Part print with two shaded views. Sizes in mm from the minimum x, y, z corner. A direction names the side the tool comes from. Coordinates: 2 decimals unless noted, no trailing zeros. Loops run counter-clockwise (first coordinate to the right, second up) from the corner with the lowest first, then second, coordinate; pieces in that order, holes last. Notation, with made-up numbers: (47.5, 21.5) -> (83.5, 21.5) arc R20 cw to (83.5, 55.5) -> close; hole circle Ø7 at (27.25, -16). An arc over 180 degrees is marked (long way). One line per item, written item: value. Start each with the question number.
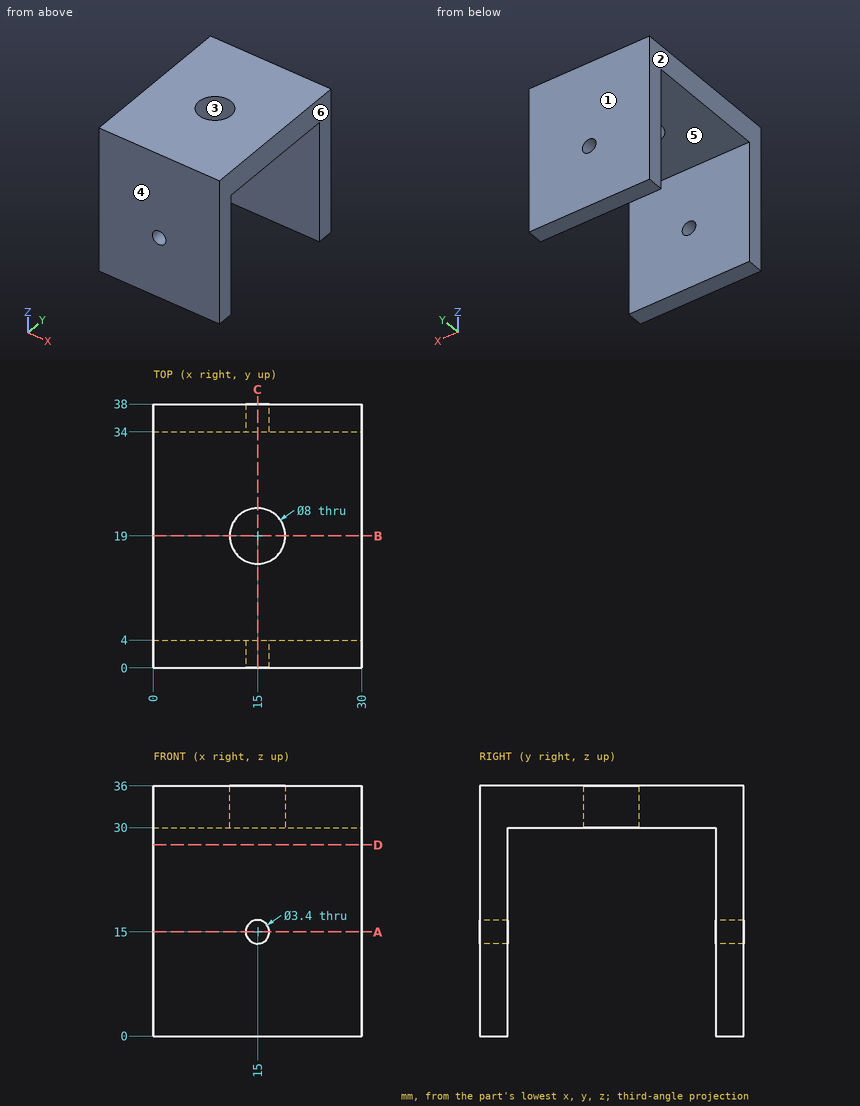
Item 1: Band-saw the part on D-D, the plane z = 27.5. List the corners of the cut face in (x, y).
Item 2: Probe probe 1 along Y at (x, z) = (14.5, 27.5); probe 2 along Z at (x, y) = (15, 36.6); probe 3 along Z at (x, y) = (5, 31.5). List the from-to ranges inside material, lowest first.
Item 3: Band-saw the part on B-B, the plane y = 19. List the corners of the cut face in (x, z).
Item 4: Band-saw the part on C-C, the plane x = 15. List the corners of the cut face in (y, z).
Item 5: Tool access for the marked faces 5 and 6: list every direction of +Z, -Z, +X, -X, +Y, -Y with a clear straight run to the whole face (end or side of a thin tool).
Item 6: Band-saw the part on A-A, the plane z = 15. List the corners of the cut face in (x, y).
Item 7: Drop a flat-ended pin along its axis: pin 1 Ø3 at (x, y) = (4, 27) entering from -Z. Give the stop position or say it passes through.
Item 8: Two-plate mould, pull along Y, no slides. Class the marked faces 1, 2, 3 and 4: +Y half, -Y half, draft (parallel to the pull), parting line (faces both ways), or undercut.
Worked out:
1. outline: (0, 0) -> (30, 0) -> (30, 4) -> (0, 4) -> close; (0, 34) -> (30, 34) -> (30, 38) -> (0, 38) -> close
2. probe 1: y = 0 to 4, 34 to 38
2. probe 2: z = 0 to 13.3, 16.7 to 36
2. probe 3: z = 30 to 36
3. outline: (0, 30) -> (11, 30) -> (11, 36) -> (0, 36) -> close; (19, 30) -> (30, 30) -> (30, 36) -> (19, 36) -> close
4. outline: (0, 0) -> (4, 0) -> (4, 13.3) -> (0, 13.3) -> close; (0, 16.7) -> (4, 16.7) -> (4, 30) -> (15, 30) -> (15, 36) -> (0, 36) -> close; (23, 30) -> (34, 30) -> (34, 16.7) -> (38, 16.7) -> (38, 36) -> (23, 36) -> close; (34, 0) -> (38, 0) -> (38, 13.3) -> (34, 13.3) -> close
5. face 5: -Z, +X, -X
5. face 6: +Z, -Z, +X, +Y, -Y
6. outline: (0, 0) -> (13.3, 0) -> (13.3, 4) -> (0, 4) -> close; (0, 34) -> (13.3, 34) -> (13.3, 38) -> (0, 38) -> close; (16.7, 0) -> (30, 0) -> (30, 4) -> (16.7, 4) -> close; (16.7, 34) -> (30, 34) -> (30, 38) -> (16.7, 38) -> close
7. pin 1: stops at z = 30
8. face 1: +Y half
8. face 2: draft
8. face 3: undercut
8. face 4: -Y half
